from build123d import *

# Parameters (mm, degrees)
EXTRUDE_1_2_DEPTH    = 1.2
EXTRUDE_16_DEPTH     = 16
EXTRUDE_32_DEPTH     = 32
SKETCH_24_138_5_W    = 4.5
SKETCH_24_138_5_H    = 24
CUT_EXTRUDE_24_DEPTH = 20
EXTRUDE_884_DEPTH    = 1.2
FILLET_R2_R          = 2


with BuildPart() as part:
    # 草图_平板外形_总宽32_舌宽16_对称过渡 → 拉伸_板厚1点2 (new body)
    with BuildSketch(Plane.XY.offset(-306.8)):
        with BuildLine():
            Line((-3.5, 122.5), (2.5, 122.5))
            add(Edge.make_bspline(
                [(2.5, 122.5), (2.568251017, 122.504680022), (2.707904652, 122.514256172), (2.913789315, 122.58691144), (3.117968932, 122.696636373), (3.321081083, 122.844952736), (3.523655529, 123.027402997), (3.725998426, 123.241623536), (3.928269446, 123.484685473), (4.130543205, 123.753813901), (4.33285106, 124.046152711), (4.53520279, 124.358837958), (4.737597952, 124.688983876), (4.940031434, 125.033693923), (5.142496177, 125.390062896), (5.344984435, 125.755180133), (5.547488324, 126.126131323), (5.75, 126.5), (5.952511676, 126.873868677), (6.155015565, 127.244819867), (6.357503823, 127.609937104), (6.559968566, 127.966306077), (6.762402048, 128.311016124), (6.96479721, 128.641162042), (7.16714894, 128.953847289), (7.369456795, 129.246186099), (7.571730554, 129.515314527), (7.774001574, 129.758376464), (7.976344471, 129.972597003), (8.178918917, 130.155047264), (8.382031068, 130.303363627), (8.586210685, 130.41308856), (8.792095348, 130.485743828), (8.931748983, 130.495319978), (9, 130.5)],
                knots=[0, 0, 0, 0, 0.019229913, 0.039347798, 0.060985216, 0.084517213, 0.110120649, 0.137834401, 0.167605027, 0.199317689, 0.232816328, 0.26791678, 0.304415434, 0.342095061, 0.380728864, 0.420083383, 0.459920669, 0.5, 0.540079331, 0.579916617, 0.619271136, 0.657904939, 0.695584566, 0.73208322, 0.767183672, 0.800682311, 0.832394973, 0.862165599, 0.889879351, 0.915482787, 0.939014784, 0.960652202, 0.980770087, 1, 1, 1, 1], degree=3))
            Line((9, 130.5), (63.2, 130.5))
            Line((63.2, 130.5), (63.2, 146.5))
            Line((63.2, 146.5), (9, 146.5))
            add(Edge.make_bspline(
                [(2.5, 154.5), (2.568251017, 154.495319978), (2.707904652, 154.485743828), (2.913789315, 154.41308856), (3.117968932, 154.303363627), (3.321081083, 154.155047264), (3.523655529, 153.972597003), (3.725998426, 153.758376464), (3.928269446, 153.515314527), (4.130543205, 153.246186099), (4.33285106, 152.953847289), (4.53520279, 152.641162042), (4.737597952, 152.311016124), (4.940031434, 151.966306077), (5.142496177, 151.609937104), (5.344984435, 151.244819867), (5.547488324, 150.873868677), (5.75, 150.5), (5.952511676, 150.126131323), (6.155015565, 149.755180133), (6.357503823, 149.390062896), (6.559968566, 149.033693923), (6.762402048, 148.688983876), (6.96479721, 148.358837958), (7.16714894, 148.046152711), (7.369456795, 147.753813901), (7.571730554, 147.484685473), (7.774001574, 147.241623536), (7.976344471, 147.027402997), (8.178918917, 146.844952736), (8.382031068, 146.696636373), (8.586210685, 146.58691144), (8.792095348, 146.514256172), (8.931748983, 146.504680022), (9, 146.5)],
                knots=[0, 0, 0, 0, 0.019229913, 0.039347798, 0.060985216, 0.084517213, 0.110120649, 0.137834401, 0.167605027, 0.199317689, 0.232816328, 0.26791678, 0.304415434, 0.342095061, 0.380728864, 0.420083383, 0.459920669, 0.5, 0.540079331, 0.579916617, 0.619271136, 0.657904939, 0.695584566, 0.73208322, 0.767183672, 0.800682311, 0.832394973, 0.862165599, 0.889879351, 0.915482787, 0.939014784, 0.960652202, 0.980770087, 1, 1, 1, 1], degree=3))
            Line((2.5, 154.5), (-3.5, 154.5))
            Line((-3.5, 154.5), (-3.5, 122.5))
        make_face()
    extrude(amount=EXTRUDE_1_2_DEPTH)

    # Sketch 429 → 拉伸_舌宽16 (add)
    with BuildSketch(Plane(origin=(0, 130.5, 0), x_dir=(1, 0, 0), z_dir=(0, 1, 0))):
        with BuildLine():
            Line((9, 306.8), (63.5, 306.8))
            Line((63.5, 306.8), (63.5, 306.723790008))
            ThreePointArc((63.5, 306.723790008), (64.58930082, 306.104776448), (65.218221983, 305.021165708))
            Line((65.218221983, 305.021165708), (66.512317209, 300.191536577))
            Line((66.512317209, 300.191536577), (65.353206217, 299.880953723))
            Line((65.353206217, 299.880953723), (64.059110992, 304.710582854))
            ThreePointArc((64.059110992, 304.710582854), (63.74465041, 305.252388224), (63.2, 305.561895004))
            Line((63.2, 305.561895004), (63.2, 305.6))
            Line((63.2, 305.6), (9, 305.6))
            Line((9, 305.6), (9, 306.8))
        make_face()
    extrude(amount=EXTRUDE_16_DEPTH)

    # Sketch 524 → 拉伸_头部总宽32 (add)
    with BuildSketch(Plane(origin=(0, 122.5, 0), x_dir=(1, 0, 0), z_dir=(0, 1, 0))):
        with BuildLine():
            Line((-5.7, 304.3), (-11.71944631, 304.3))
            Line((-11.71944631, 304.3), (-11.71944631, 303.1))
            Line((-11.71944631, 303.1), (-5.7, 303.1))
            ThreePointArc((-5.7, 303.1), (-4.497918472, 303.597918472), (-4, 304.8))
            Line((-4, 304.8), (-4, 305.1))
            ThreePointArc((-4, 305.1), (-3.853553391, 305.453553391), (-3.5, 305.6))
            Line((-3.5, 305.6), (2.5, 305.6))
            Line((2.5, 305.6), (2.5, 306.8))
            Line((2.5, 306.8), (-3.5, 306.8))
            ThreePointArc((-3.5, 306.8), (-4.702081528, 306.302081528), (-5.2, 305.1))
            Line((-5.2, 305.1), (-5.2, 304.8))
            ThreePointArc((-5.2, 304.8), (-5.346446609, 304.446446609), (-5.7, 304.3))
        make_face()
    extrude(amount=EXTRUDE_32_DEPTH)

    # 草图_榫槽净宽24_中线138点5 → 切除_榫槽24 (cut)
    with BuildSketch(Plane.XY.offset(-299)):
        with Locations((-5.75, 138.5)):
            Rectangle(SKETCH_24_138_5_W, SKETCH_24_138_5_H)
    extrude(amount=-CUT_EXTRUDE_24_DEPTH, mode=Mode.SUBTRACT)

    # 草图_头部完整外形_总宽32_槽24 → Extrude 884 (add)
    with BuildSketch(Plane.XY.offset(-304.3)):
        with BuildLine():
            Line((-5.7, 154.5), (-5.7, 150.5))
            Line((-5.7, 150.5), (-8, 150.5))
            Line((-8, 150.5), (-8, 126.5))
            Line((-8, 126.5), (-5.7, 126.5))
            Line((-5.7, 126.5), (-5.7, 122.5))
            Line((-5.7, 122.5), (-11.71944631, 122.5))
            add(Edge.make_bspline(
                [(-12.5, 124.034562212), (-12.499938159, 124.023029786), (-12.499814468, 123.999963286), (-12.498936319, 123.965367365), (-12.497443181, 123.93078278), (-12.495403218, 123.896208954), (-12.492747447, 123.861654709), (-12.489510446, 123.827122022), (-12.485676021, 123.792616625), (-12.481245518, 123.758142921), (-12.476215317, 123.723705745), (-12.47058192, 123.689310059), (-12.464341601, 123.654960897), (-12.457490017, 123.620663481), (-12.450022451, 123.586423185), (-12.441933692, 123.552245581), (-12.433218056, 123.518136449), (-12.423869366, 123.484101803), (-12.413880931, 123.450147918), (-12.403245533, 123.416281356), (-12.391955405, 123.382508994), (-12.380002212, 123.348838059), (-12.367377024, 123.31527616), (-12.354070301, 123.281831329), (-12.340071858, 123.248512061), (-12.325370845, 123.215327364), (-12.309955716, 123.182286805), (-12.293814204, 123.149400568), (-12.276933286, 123.116679519), (-12.259299156, 123.08413527), (-12.240897191, 123.05178026), (-12.221711924, 123.019627836), (-12.201727007, 122.987692349), (-12.180925191, 122.955989258), (-12.159288292, 122.92453525), (-12.136797175, 122.893348363), (-12.113431735, 122.862448139), (-12.089170893, 122.831855779), (-12.063992595, 122.801594323), (-12.037873835, 122.771688857), (-12.010790698, 122.742166721), (-11.982718406, 122.713057784), (-11.953631496, 122.684394601), (-11.923503642, 122.656213171), (-11.892309147, 122.628551369), (-11.860018463, 122.601456324), (-11.826614179, 122.574961378), (-11.792043997, 122.549159388), (-11.756366816, 122.523975845), (-11.731804684, 122.508025417), (-11.71944631, 122.5)],
                knots=[0, 0, 0, 0, 0.019280259, 0.038563274, 0.057853041, 0.077151606, 0.096462833, 0.115789535, 0.135134996, 0.15450244, 0.173895129, 0.193316406, 0.212769662, 0.232258368, 0.251786071, 0.271356411, 0.290973123, 0.310640051, 0.330361155, 0.350140527, 0.369982395, 0.389891141, 0.409871307, 0.429927615, 0.450064974, 0.4702885, 0.490603526, 0.511015624, 0.531530615, 0.552154592, 0.572893933, 0.593755326, 0.61474578, 0.635872653, 0.657143665, 0.678566916, 0.700150912, 0.721904572, 0.743837244, 0.765958718, 0.788279226, 0.81080944, 0.83356046, 0.856543784, 0.879771256, 0.903255123, 0.927007303, 0.951041228, 0.97536652, 1, 1, 1, 1], degree=3))
            Line((-12.5, 124.034562212), (-12.5, 152.965437788))
            add(Edge.make_bspline(
                [(-11.71944631, 154.5), (-11.731804684, 154.491974583), (-11.756366816, 154.476024155), (-11.792043997, 154.450840612), (-11.826614179, 154.425038622), (-11.860018463, 154.398543676), (-11.892309147, 154.371448631), (-11.923503642, 154.343786829), (-11.953631496, 154.315605399), (-11.982718406, 154.286942216), (-12.010790698, 154.257833279), (-12.037873835, 154.228311143), (-12.063992595, 154.198405677), (-12.089170893, 154.168144221), (-12.113431735, 154.137551861), (-12.136797175, 154.106651637), (-12.159288292, 154.07546475), (-12.180925191, 154.044010742), (-12.201727007, 154.012307651), (-12.221711924, 153.980372164), (-12.240897191, 153.94821974), (-12.259299156, 153.91586473), (-12.276933286, 153.883320481), (-12.293814204, 153.850599432), (-12.309955716, 153.817713195), (-12.325370845, 153.784672636), (-12.340071858, 153.751487939), (-12.354070301, 153.718168671), (-12.367377024, 153.68472384), (-12.380002212, 153.651161941), (-12.391955405, 153.617491006), (-12.403245533, 153.583718644), (-12.413880931, 153.549852082), (-12.423869366, 153.515898197), (-12.433218056, 153.481863551), (-12.441933692, 153.447754419), (-12.450022451, 153.413576815), (-12.457490017, 153.379336519), (-12.464341601, 153.345039103), (-12.47058192, 153.310689941), (-12.476215317, 153.276294255), (-12.481245518, 153.241857079), (-12.485676021, 153.207383375), (-12.489510446, 153.172877978), (-12.492747447, 153.138345291), (-12.495403218, 153.103791046), (-12.497443181, 153.06921722), (-12.498936319, 153.034632635), (-12.499814468, 153.000036714), (-12.499938159, 152.976970214), (-12.5, 152.965437788)],
                knots=[0, 0, 0, 0, 0.02463348, 0.048958772, 0.072992697, 0.096744877, 0.120228744, 0.143456216, 0.16643954, 0.18919056, 0.211720774, 0.234041282, 0.256162756, 0.278095428, 0.299849088, 0.321433084, 0.342856335, 0.364127347, 0.38525422, 0.406244674, 0.427106067, 0.447845408, 0.468469385, 0.488984376, 0.509396474, 0.5297115, 0.549935026, 0.570072385, 0.590128693, 0.610108859, 0.630017605, 0.649859473, 0.669638845, 0.689359949, 0.709026877, 0.728643589, 0.748213929, 0.767741632, 0.787230338, 0.806683594, 0.826104871, 0.84549756, 0.864865004, 0.884210465, 0.903537167, 0.922848394, 0.942146959, 0.961436726, 0.980719741, 1, 1, 1, 1], degree=3))
            Line((-11.71944631, 154.5), (-5.7, 154.5))
        make_face()
    extrude(amount=EXTRUDE_884_DEPTH)

    # 圆角_舌片上下端角_R2
    fillet_r2_edges = [part.edges().sort_by_distance(p)[0] for p in [
        (65.932761713, 146.5, -300.03624515),
        (65.932761713, 130.5, -300.03624515),
    ]]
    fillet(fillet_r2_edges, radius=FILLET_R2_R)


solid = part.part
Input: part model. Units: mm. Frame: model coordinates. A direction names the side the tool comes from. Give positions to 0.01 mm unless a question says otherwise; leave off trailing zeros. Write each loop counter-clockwise with the first axis right and the second up, starting at its lowest first coordinate (ties: lowest second). Pieces come first, ordered by that corner, then holes. Notation, with made-up numbers: (72.5, 89.5) -> (124.5, 89.5) arc R11 ccw to (124.5, 93.5) -> close; hole circle Ø6 at (-34, 77.5). An arc over 180 degrees is marked (long way). Use one line per item in the form item = value. Start each with the question number.
1) Pin query (flat end, axial travel): pin 1 (7.5 mm diameter, centred on x = -9.5, y = 130.5, fed in from -Z); pin 2 (2.5 mm diameter, centred on x = 25.5, z = -305, fed in from -Y); pin 3 (5.5 mm diameter, centred on x = -9.5, y = 133.5, fed in from +Z). Return the tip coordinate at first contact, or that it passes through.
2) Section query B-B on x = -2. Return the cut outline in (y, z).
3) Section query C-C on x = 47. Return the cut outline in (y, z).
4) Ray query, probe 1 along Z at (x, y) = (15.5, 139.5); probe 2 along X at (y, z) = (147.5, -303.25); probe 3 along Y at (x, z) = (34, -306). Return the intervals inside material, ascending. Write a range as from..to.
5) Set-up query: faces 1 (the cylindrical face through (64.577, 138.388, -306.117)), 2 (the flat face through (-10, 138, -304.3)), 3 (the flat face through (-10, 138, -303.1)), 4 (the flat face through (64.715, 138.388, -302.262)). Return all of +Z, -Z, +X, -X, +Y, -Y with unobstructed straight access to the full face (end or side cutting, diameter ignored); none if empty.
6) Draft query along Y for faces 5 (the flat face through (40, 146.5, -306)), 6 (the flat face through (-5, 150.5, -305)), 7 (the flat face through (39, 130.5, -306)). Return one class per face: pulls with the +Y half, pulls with the -Y half, needs draft (parallel to the pull), parting line crosses it, or undercut.
Outcome:
q1.pin_1 = -304.3
q1.pin_2 = 130.5
q1.pin_3 = -303.1
q2.outline = (122.5, -306.8) -> (154.5, -306.8) -> (154.5, -305.6) -> (122.5, -305.6) -> close
q3.outline = (130.5, -306.8) -> (146.5, -306.8) -> (146.5, -305.6) -> (130.5, -305.6) -> close
q4.probe_1 = -306.8..-305.6
q4.probe_2 = -12.5..-8
q4.probe_3 = 130.5..146.5
q5.face_1 = -Z, +X, +Y, -Y
q5.face_2 = -Z, -X, +Y, -Y
q5.face_3 = +Z, -X, +Y, -Y
q5.face_4 = +Z, +Y, -Y
q6.face_5 = pulls with the +Y half
q6.face_6 = undercut
q6.face_7 = pulls with the -Y half
